Source: three-view drawing plus pictorial views. Frame: mm from the lowest corner of the part. A direction names the side the tool comes from. Give positions to 0.01 mm unless a question says otherwise; leave off trailing zeros. Order: outer loops, then holes, each group sorted by start corner. A loop starts at its lowest first (then second) coordinate and runs counter-clockwise, first axis right, second up. Notation, with made-up numbers: (-20, 27.5) -> (-8, 27.5) arc R18 cw to (-8, 38.5) -> close; hole circle Ø3 at (-6.75, 9.5). An arc over 180 degrees is marked (long way). Answer in a Markdown table with one row per item. Add a question column.
Q1. Cut plane C-C on x = 75. Return the cut outline in (y, z), and give its area (3 significant figures).
Q2. Cut plane B-B on z = 21. Return the cut outline in (x, y) (1 decimal).
Q3. Contact query for flat-ended pins moving along their axis: P1, Ø10, axis at x = 75.5, z = 20.5, coming from the -Y side; P2, Ø3, axis at x = 13.5, z = 5.5, coming from the -Y side; P3, Ø13, axis at y = 75.5, z = 27.5, coming from the +X side; P4, Ø6, axis at x = 38, z = 42.5, coming from the +Y side. Output: stop coordinate, or through.
Q4. Pull-direction query (Z, two-part tool) for the marked faces 4, 5, 6 and 7; classes: +Z half, -Z half, draft (parallel to the pull), parting line (faces both ways), or undercut.
Q5. Set-up query: the marked faces 1, 2 and 3. Return all of +Z, -Z, +X, -X, +Y, -Y with unobstructed straight access to the full face (end or side cutting, diameter ignored); none if empty.
Q6. Cut plane A-A on y = 30.5. Return the cut outline in (x, z) (1 decimal), and give its area (3 significant figures).
Q7. Line query: line 1 along X through (y, z) = (17, 43) (1 decimal); line 2 along Y through (x, z) = (55, 21.5); line 3 along Y through (x, z) = (73, 9). Output: solid intervals per line, ascending. Write a range as from..to.
Q8. Cut plane D-D on z = 46. Return the cut outline in (x, y) (1 decimal).
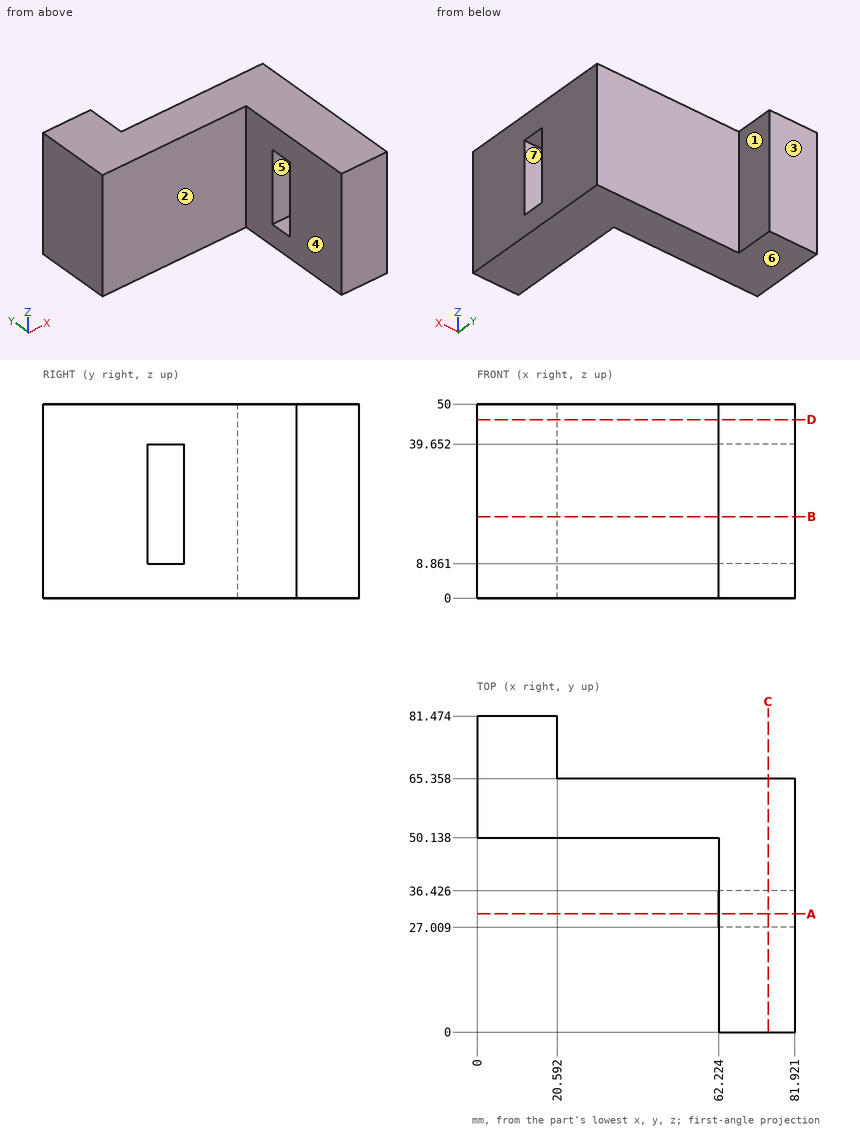
Completed:
| question | item | result |
|---|---|---|
| 1 | outline | (0, 0) -> (65.36, 0) -> (65.36, 50) -> (0, 50) -> close; hole (27.01, 8.86) -> (36.43, 8.86) -> (36.43, 39.65) -> (27.01, 39.65) -> close |
| 1 | area | 2,980 mm² |
| 2 | outline | (0, 50.1) -> (62.2, 50.1) -> (62.2, 36.4) -> (81.9, 36.4) -> (81.9, 65.4) -> (20.6, 65.4) -> (20.6, 81.5) -> (0, 81.5) -> close; (62.2, 0) -> (81.9, 0) -> (81.9, 27) -> (62.2, 27) -> close |
| 3 | P1 | stops at y = 0 |
| 3 | P2 | stops at y = 50.14 |
| 3 | P3 | stops at x = 20.59 |
| 3 | P4 | stops at y = 65.36 |
| 4 | face 4 | draft |
| 4 | face 5 | undercut |
| 4 | face 6 | -Z half |
| 4 | face 7 | undercut |
| 5 | face 1 | +Z, -Z, +X, +Y |
| 5 | face 2 | +Z, -Z, -X, -Y |
| 5 | face 3 | +Z, -Z, +X, -X, +Y |
| 6 | outline | (62.2, 0) -> (81.9, 0) -> (81.9, 8.9) -> (62.2, 8.9) -> close; (62.2, 39.7) -> (81.9, 39.7) -> (81.9, 50) -> (62.2, 50) -> close |
| 6 | area | 378 mm² |
| 7 | line 1 | x = 62.2..81.9 |
| 7 | line 2 | y = 50.14..65.36 |
| 7 | line 3 | y = 0..27.01, 36.43..65.36 |
| 8 | outline | (0, 50.1) -> (62.2, 50.1) -> (62.2, 0) -> (81.9, 0) -> (81.9, 65.4) -> (20.6, 65.4) -> (20.6, 81.5) -> (0, 81.5) -> close |
